```python
from build123d import *

# Parameters (mm, degrees)
F1_DEPTH = 38.1
F2_R     = 12.7
F2_R_2   = 9.525
F3_DEPTH = 6.35


# Not quite as in the source:
# - a feature names something its author has since deleted; it is built from what else it names


with BuildPart() as f1:
    # F0 (on Right) → F1 (new body)
    with BuildSketch(Plane.YZ):
        Polygon((-31.75, 0), (0, 0), (31.75, 0), (31.75, 12.7), (19.05, 12.7), (19.05, 25.4), (-19.05, 25.4), (-19.05, 12.7), (-31.75, 12.7), align=None)
    extrude(amount=F1_DEPTH)

    # F2 (on face) → F3 (join)
    with BuildSketch(Plane.XY.offset(25.4)):
        with Locations((19.05, 0)):
            Circle(F2_R)
        with Locations((19.05, 0)):
            Circle(F2_R_2, mode=Mode.SUBTRACT)
    extrude(amount=F3_DEPTH)


solid = f1.part
```
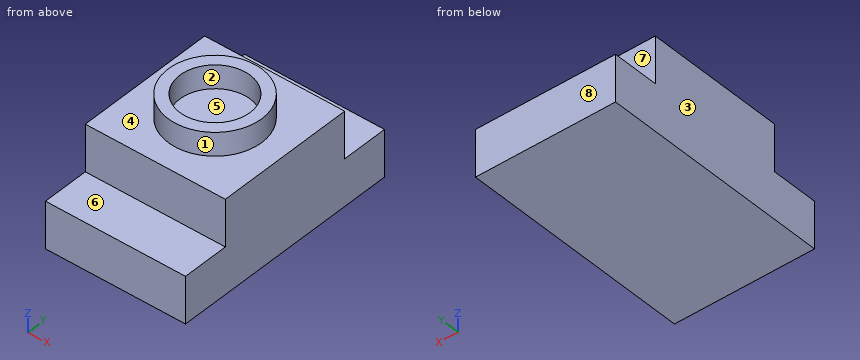
The listing builds one solid part. Answer for the finished solid, in the listing's coordinates (mm). Face numbers are marked on the shaded views. A direction names the side the tool comes from. Give positions to 0.01 mm unless a question says otherwise; leave off trailing zeros. Order: outer loops, then holes, each group sorted by start corner. A loop starts at its lowest first (then second) coordinate and runs counter-clockwise, first axis right, second up. Notation, with made-up numbers: (6.25, 38.25) - (19.25, 38.25) arc R14 cw to (19.25, 59.25) - close; hole circle Ø10 at (22.25, 53.5). An arc over 180 degrees is marked (long way). Use one line per item in the form item = value. Start each with the question number.
(1) A cutting plane is placed at B-B, the plane y = 0. Write down the section's boundary in (x, z) (3 decimals).
(2) A cutting plane is placed at A-A, the plane x = 36. Write down the section's boundary in (y, z).
(3) The mould has two halves that part along X. Classify the marked faces 1, 2, 3 and 4: released by +X, released by -X, zero draft, split by the parting line, or undercut.
(4) Consider line 1 (Y direction, x = 19.05, z = 29.5) (3 decimals); line 2 (Z direction, x = 34.5, y = -24); line 3 (Z direction, x = 34, y = 15). Determine where each line is inside the solid, lowest interval first. Write a range as from..to.
(5) A cutting plane is placed at C-C, the plane x = 19.05. Write down the section's boundary in (y, z) (3 decimals), then the cut area to 3 significant figures.
(6) Flat-ended cylindrical pins translate along their axes: pin 1 Ø10 at (x, y) = (18.5, 27.5) entering from +Z; pin 2 Ø6.5 at (x, z) = (26.5, 17.5) entering from -Y; pin 3 Ø5.5 at (x, y) = (20, 0) entering from +Z. Find the tip coordinate at first contact, or state that the pin passes through.
(7) A cutting plane is placed at D-D, the plane z = 18. Write down the section's boundary in (x, y), then the cut area to 3 significant figures.
(8) For the marked faces 5, 6, 7 and 8, determine the directions among +Z, -Z, +X, -X, +Y, -Y from which every point of the face is accessible in a straight line to the end or side of a thin tool.
Ans:
q1.outline = (0, 0) - (38.1, 0) - (38.1, 25.4) - (31.75, 25.4) - (31.75, 31.75) - (28.575, 31.75) - (28.575, 25.4) - (9.525, 25.4) - (9.525, 31.75) - (6.35, 31.75) - (6.35, 25.4) - (0, 25.4) - close
q2.outline = (-31.75, 0) - (31.75, 0) - (31.75, 12.7) - (19.05, 12.7) - (19.05, 25.4) - (-19.05, 25.4) - (-19.05, 12.7) - (-31.75, 12.7) - close
q3.face_1 = split by the parting line
q3.face_2 = undercut
q3.face_3 = released by -X
q3.face_4 = zero draft
q4.line_1 = -12.7..-9.525, 9.525..12.7
q4.line_2 = 0..12.7
q4.line_3 = 0..25.4
q5.outline = (-31.75, 0) - (31.75, 0) - (31.75, 12.7) - (19.05, 12.7) - (19.05, 25.4) - (12.7, 25.4) - (12.7, 31.75) - (9.525, 31.75) - (9.525, 25.4) - (-9.525, 25.4) - (-9.525, 31.75) - (-12.7, 31.75) - (-12.7, 25.4) - (-19.05, 25.4) - (-19.05, 12.7) - (-31.75, 12.7) - close
q5.area = 1,330 mm^2
q6.pin_1 = 12.7
q6.pin_2 = -19.05
q6.pin_3 = 25.4
q7.outline = (0, -19.05) - (38.1, -19.05) - (38.1, 19.05) - (0, 19.05) - close
q7.area = 1,450 mm^2
q8.face_5 = +Z
q8.face_6 = +Z, +X, -X, -Y
q8.face_7 = +Z, +X, -X, +Y
q8.face_8 = +Z, -Z, +X, -X, +Y
